Geometry check sheet. Reference: the model listing, model coordinates, mm. A direction names the side the tool comes from. Round coordinates to 2 decimals unless told otherwise and drop trailing zeros. Write each loop counter-clockwise with the first axis right and the second up, starting at its lowest first coordinate (ties: lowest second). Pieces come first, ordered by that corner, then holes. Notation, with made-up numbers: M -22,60 L 6,60 A15 ccw 6,77 Z; hole C 3,21.5 d3. An arc over 180 degrees is marked long. One line per item, written item: value. Start each with the question number.
1. Section check A-A (y = 4.5). Record the boundary of the cut face in (x, z).
2. Section check C-C (x = -3.5). Record the boundary of the cut face in (y, z).
3. Release check for a two-part mould opening along X. For faces 6 (the flat face through (-0.27, -7.16, 41.81)), 7 (the flat face through (-1, -32, 17)), 8 (the flat face through (-32, 0, 42)) record: pulls with the +X half, pulls with the -X half, needs draft (parallel to the pull), parting line crosses it, or undercut.
4. Section check D-D (x = -48.5). Record the boundary of the cut face in (y, z), and give its area (3 significant figures).
5. Scan lines: probe 1 along X at (y, z) = (0, 6.5); probe 2 along X at (y, z) = (-10.5, 58); probe 3 along Y at (x, z) = (57, 10.5). Record each from-to range of solid material in increasing order. Write a range as [from, to].
6. Access from +Z, -Z, +X, -X, +Y, -Y to the whole of each face (thin tool, end or side, straight path). Record for faces 1 (the flat face through (-67, 8, 19)), 2 (the flat face through (32, 0, 42)), 3 (the flat face through (-19, -18, 52)), 4 (the flat face through (1, 32, 24)), 5 (the cylindrical face through (46, 0, 9)).
7. Section check B-B (z = 7.5). Record the boundary of the cut face in (x, y).
8. Depth check by flat-ended pin: P1, Ø22.5, axis at y = 10, z = 32, coming from the +X side; P2, Ø2, axis at y = 25.5, z = 18.5, coming from the -X side; P3, Ø2, axis at x = -11, z = 52, coming from the -Y side. Enter the tip coordinate at first touch or a pass-through.
Autodesk Fusion 360 part; units mm, degrees
sketch "Sketch1" plane through (0, 0, 0) normal (0, 0, 1) x (1, 0, 0)
  line L0 (57, 32) -> (-57, 32)
  line L1 (-57, 32) -> (-57, -32)
  line L2 (-57, -32) -> (57, -32)
  line L3 (57, -32) -> (57, 32)
  line L4 (57, 32) -> (-57, -32) construction
  line L5 (-57, 32) -> (57, -32) construction
  line L6 (-32, 32) -> (-32, -32) construction
  line L7 (32, 32) -> (32, -32) construction
  circle A0 centre (57, 0) radius 11
  circle A1 centre (-57, 0) radius 11
  circle A2 centre (-57, 0) radius 32
  circle A3 centre (57, 0) radius 32
  dimension "d1" = 114
  dimension "d2" = 64
  dimension "d3" = 64
  dimension "d4" = 25
  dimension "d5" = 22
  dimension "d6" = 22
  dimension "d7" = 32
  dimension "d8" = 32
extrude "Extrude1" add sketch "Sketch1" along normal blind 19 contours L0 L2 A2 A3 | L3 A0 A3 | L3 A0 A3 | L1 A1 A2 | L1 A1 A2
sketch "Sketch2" plane through (0, 0, 0) normal (1, 0, 0) x (0, 1, 0)
  line L0 (-32, 19) -> (32, 19)
  line L1 (32, 19) -> (32, 64)
  line L2 (32, 64) -> (17, 64)
  line L3 (17, 64) -> (-32, 19)
  dimension "d11" = 45
  dimension "d13" = 15
extrude "Extrude2" add sketch "Sketch2" along normal mid plane 38
sketch "Sketch3" plane through (19, 0, 0) normal (1, 0, 0) x (0, 1, 0)
  line L0 (17, 64) -> (-32, 19)
  line L1 (-32, 19) -> (32, 19)
  line L2 (32, 19) -> (32, 64)
  line L3 (32, 64) -> (17, 64)
  line L4 (-32, 19) -> (32, 19)
  line L5 (32, 19) -> (32, 64)
  line L6 (32, 64) -> (-32, 64)
  line L7 (-32, 64) -> (-32, 19)
extrude "Extrude3" add sketch "Sketch3" along normal blind 13
sketch "Sketch4" plane through (-19, 0, 0) normal (-1, 0, 0) x (0, -1, 0)
  line L0 (32, 19) -> (-17, 64)
  line L1 (-17, 64) -> (-32, 64)
  line L2 (-32, 64) -> (-32, 19)
  line L3 (-32, 19) -> (32, 19)
  line L4 (-32, 64) -> (32, 64)
  line L5 (32, 64) -> (32, 19)
  line L6 (32, 19) -> (-32, 19)
  line L7 (-32, 64) -> (-32, 19)
extrude "Extrude4" add sketch "Sketch4" along normal blind 13
Result sheet:
1. outline: M -88.68,0 L -67.04,0 L -67.04,19 L -88.68,19 Z; M -46.96,0 L 46.96,0 L 46.96,19 L 32,19 L 32,64 L 19,64 L 19,52.52 L -19,52.52 L -19,64 L -32,64 L -32,19 L -46.96,19 Z; M 67.04,0 L 88.68,0 L 88.68,19 L 67.04,19 Z
2. outline: M -32,0 L 32,0 L 32,64 L 17,64 L -32,19 Z
3. face 6: undercut
3. face 7: needs draft
3. face 8: pulls with the -X half
4. outline: M -32,0 L -6.98,0 L -6.98,19 L -32,19 Z; M 6.98,0 L 32,0 L 32,19 L 6.98,19 Z
4. area: 951 mm2
5. probe 1: x = [-89, -68], [-46, 46], [68, 89]
5. probe 2: x = [-32, -19], [19, 32]
5. probe 3: y = [-32, -11], [11, 32]
6. face 1: +Z, -X, +Y, -Y
6. face 2: +Z, +X, +Y, -Y
6. face 3: +Z, -Y
6. face 4: +Z, -Z, +X, -X, +Y
6. face 5: +Z, -Z
7. outline: M -57,-32 L 57,-32 A32 ccw 57,32 L -57,32 A32 ccw Z; hole C -57,0 d22; hole C 57,0 d22
8. P1: stops at x = 32
8. P2: stops at x = -77.59
8. P3: stops at y = 2.84
